from build123d import *

# Parameters (mm, degrees)
SKETCH1_W           = 650
SKETCH1_H           = 200
SKETCH1_W_2         = 500
SKETCH1_H_2         = 15
SKETCH1_W_3         = 10
SKETCH1_H_3         = 20
BOSS_EXTRUDE1_DEPTH = 20
SKETCH2_W           = 10
SKETCH2_H           = 10
BOSS_EXTRUDE2_DEPTH = 20


with BuildPart() as part:
    # Sketch1 → Boss-Extrude1 (new body)
    with BuildSketch(Plane.XY):
        Rectangle(SKETCH1_W, SKETCH1_H)
        Rectangle(SKETCH1_W_2, SKETCH1_H_2, mode=Mode.SUBTRACT)
        with Locations((-290, 0)):
            Rectangle(SKETCH1_W_3, SKETCH1_H_3, mode=Mode.SUBTRACT)
        with Locations((290, 0)):
            Rectangle(SKETCH1_W_3, SKETCH1_H_3, mode=Mode.SUBTRACT)
    extrude(amount=BOSS_EXTRUDE1_DEPTH)

    # Sketch2 → Boss-Extrude2 (add)
    with BuildSketch(Plane(origin=(0, 100, 0), x_dir=(1, 0, 0), z_dir=(0, 1, 0))):
        with Locations((-180, -10)):
            Rectangle(SKETCH2_W, SKETCH2_H)
        with Locations((-220, -10)):
            Rectangle(SKETCH2_W, SKETCH2_H)
        with Locations((-140, -10)):
            Rectangle(SKETCH2_W, SKETCH2_H)
        with Locations((-100, -10)):
            Rectangle(SKETCH2_W, SKETCH2_H)
        with Locations((-60, -10)):
            Rectangle(SKETCH2_W, SKETCH2_H)
        with Locations((-20, -10)):
            Rectangle(SKETCH2_W, SKETCH2_H)
        with Locations((20, -10)):
            Rectangle(SKETCH2_W, SKETCH2_H)
        with Locations((60, -10)):
            Rectangle(SKETCH2_W, SKETCH2_H)
        with Locations((100, -10)):
            Rectangle(SKETCH2_W, SKETCH2_H)
        with Locations((140, -10)):
            Rectangle(SKETCH2_W, SKETCH2_H)
        with Locations((180, -10)):
            Rectangle(SKETCH2_W, SKETCH2_H)
        with Locations((220, -10)):
            Rectangle(SKETCH2_W, SKETCH2_H)
    extrude(amount=BOSS_EXTRUDE2_DEPTH)


solid = part.part
Geometry check sheet. Reference: the model listing, model coordinates, mm. A direction names the side the tool comes from. Round coordinates to 2 decimals unless told otherwise and drop trailing zeros. Loops run counter-clockwise (first coordinate to the right, second up) from the corner with the lowest first, then second, coordinate; pieces in that order, holes last.
Item 1: Mould release check, pull along Y, two halves, no side actions. Record for faces 1 (the flat face through (-3, 7.5, 10)), 2 (the flat face through (325, -1, 10)), 3 (the flat face through (-5, -100, 10)): pulls with the +Y half, pulls with the -Y half, needs draft (parallel to the pull), parting line crosses it, or undercut.
Item 2: Cross-section at A-A on x = -32. Record the boundary of the cut face in (y, z), then the cut area to 3 significant figures.
Item 3: Thickness scan on line 1 (X direction, y = -6, z = 13.75); line 2 (X direction, y = -9, z = 16.5); line 3 (Y direction, x = 112, z = 5). Record the ranges inside material, lowest first.
Item 4: Cross-section at B-B on z = 10.25. Count the separate pieces of the cut face and the enclosed holes in it, then the cut area to 4 significant figures.
Item 5: Access from +Z, -Z, +X, -X, +Y, -Y to the whole of each face (thin tool, end or side, straight path). Record for faces 4 (the flat face through (285, 0, 10)), 5 (the flat face through (-5, 24, 0)).
Item 6: Cross-section at C-C on x = -269. Record the boundary of the cut face in (y, z).
Item 7: Gauge pin test, flat ends, axial feed: pin 1 (11 mm diameter, centred on y = 105, z = 12, fed in from -X); pin 2 (3 mm diameter, centred on x = 182, y = 111, fed in from -Z); pin 3 (8 mm diameter, centred on y = 108, z = 12.5, fed in from -X); pin 4 (5 mm diameter, centred on x = -182, y = 105, fed in from +Z). Record the tip position at first contact, or that the pin passes through.
Answer sheet:
1. face 1: undercut
1. face 2: needs draft
1. face 3: pulls with the -Y half
2. outline: (-100, 0) - (-7.5, 0) - (-7.5, 20) - (-100, 20) - close; (7.5, 0) - (100, 0) - (100, 20) - (7.5, 20) - close
2. area: 3,700 mm2
3. line 1: x = -325 to -295, -285 to -250, 250 to 285, 295 to 325
3. line 2: x = -325 to -295, -285 to 285, 295 to 325
3. line 3: y = -100 to -7.5, 7.5 to 100
4. separate pieces: 1
4. enclosed holes: 3
4. area: 124,500 mm2
5. face 4: +Z, -Z
5. face 5: -Z, +X, -X, +Y, -Y
6. outline: (-100, 0) - (100, 0) - (100, 20) - (-100, 20) - close
7. pin 1: stops at x = -325
7. pin 2: stops at z = 5
7. pin 3: stops at x = -225
7. pin 4: stops at z = 15
